Check sheet for the modelled part. Datum: model origin and axes. Units: mm. A direction names the side the tool comes from. Coordinates: 2 decimals unless noted, no trailing zeros. Loops run counter-clockwise (first coordinate to the right, second up) from the corner with the lowest first, then second, coordinate; pieces in that order, holes last. Notation, with made-up numbers: M 70.5,65 L 74.5,65 A17 ccw 74.5,88 Z; hole C 43,6.5 d5. An arc over 180 degrees is marked long. Write each question's results on one line, items separated by ' | '. Start each with the question number.
from build123d import *

# Parameters (mm, degrees)
SKETCH1_R           = 50.5
BOSS_EXTRUDE1_DEPTH = 1
CUT_EXTRUDE1_DEPTH  = 1
CIRPATTERN1_COUNT   = 3


with BuildPart() as part:
    # Sketch1 → Boss-Extrude1 (new, symmetric)
    with BuildSketch(Plane(origin=(0, 0, 0), x_dir=(1, 0, 0), z_dir=(0, 1, 0))):
        with Locations(Location((0, 0, 0), (0, 0, 270))):
            Circle(SKETCH1_R)
    extrude(amount=BOSS_EXTRUDE1_DEPTH, both=True)

    # Sketch2 → Cut-Extrude1 (cut)
    with BuildSketch(Plane(origin=(0, 1, 0), x_dir=(1, 0, 0), z_dir=(0, 1, 0))):
        with BuildLine():
            ThreePointArc((10.381410523, 46.827516727), (0, 47.96446609), (-10.381410523, 46.827516727))
            ThreePointArc((-10.381410523, 46.827516727), (-13.040907899, 42.652942054), (-8.866333226, 39.993444677))
            ThreePointArc((-8.866333226, 39.993444677), (0, 40.96446609), (8.866333226, 39.993444677))
            ThreePointArc((8.866333226, 39.993444677), (13.040907899, 42.652942054), (10.381410523, 46.827516727))
        make_face()
    cut_extrude1 = extrude(amount=-CUT_EXTRUDE1_DEPTH, mode=Mode.SUBTRACT)

    # CirPattern1: Cut-Extrude1 ×3 about axis
    cirpattern1_axis = Axis((0, 0, 0), (0, 1, 0))
    for i in range(1, CIRPATTERN1_COUNT):
        add(cut_extrude1.rotate(cirpattern1_axis, i * 360 / CIRPATTERN1_COUNT), mode=Mode.SUBTRACT)


solid = part.part
Item 1: Section check B-B (y = -0.65). Record the cut outline in (x, z), plus the area to 3 significant figures.
Item 2: Depth check by flat-ended pin: P1, Ø1, axis at y = 0, z = -5, coming from the +X side. Enter the tip coordinate at first touch or a pass-through.
Item 3: Section check D-D (x = 22.5). Record the cut outline in (y, z), plus the area to 3 significant figures.
Item 4: Section check A-A (x = 0). Record the cut outline in (y, z).
Item 5: Thickness scan on line 1 (Z direction, x = 1, y = 0.4); line 2 (X direction, y = -0.7, z = 32); line 3 (X direction, y = 0.5, z = 28.5). Record the ranges inside material, lowest first.
Item 6: Release check for a two-part mould opening along X. For faces 1 (the face through (43.532, 0.507, 10.057)), 2 (the face through (-30.728, 0.014, -40.075)), 3 (the face through (1, 1, -1)) record: +X half, -X half, draft (parallel to the pull), parting line (faces both ways), or undercut.
Item 7: Tool access check on faces 4 (the face through (-38, 0, 22)), 5 (the face through (1, -1, -1)). Record the directions out of +Z, -Z, +X, -X, +Y, -Y that give a thin tool (end or side, any length) a straight path to the whole face; none if there is none.
Item 8: Section check C-C (z = 36.5). Record the cut outline in (x, y), plus the area to 3 significant figures.
Computed values:
1) outline: C 0,0 d101 | area: 8,010 mm²
2) P1: stops at x = 50.3
3) outline: M -1,-45.21 L 1,-45.21 L 1,45.21 L -1,45.21 Z | area: 181 mm²
4) outline: M -1,-50.5 L 1,-50.5 L 1,-47.96 L 0,-47.96 L 0,-40.96 L 1,-40.96 L 1,50.5 L -1,50.5 Z
5) line 1: z = -50.49 to -47.95, -40.95 to 50.49 | line 2: x = -39.07 to 39.07 | line 3: x = -41.69 to -38.58, -29.64 to 29.64, 38.58 to 41.69
6) face 1: undercut | face 2: parting line | face 3: draft
7) face 4: +Y | face 5: +Z, -Z, +X, -X, -Y
8) outline: M -34.9,-1 L 34.9,-1 L 34.9,1 L -34.9,1 Z | area: 140 mm²
